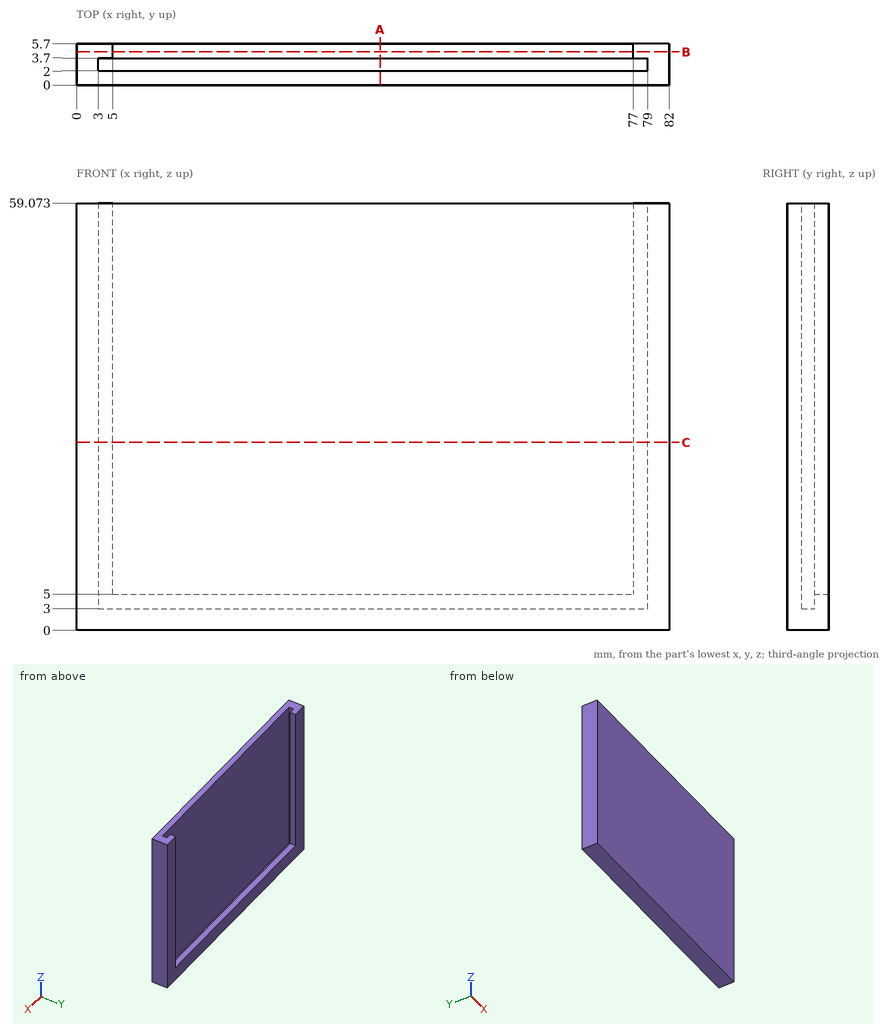
Input: dimensioned drawing with shaded views. Units: mm. Origin: part minimum x, y, z. Coordinates: 2 decimals unless noted, no trailing zeros. Order: outer loops, then holes, each group sorted by start corner. A loop starts at its lowest first (then second) coordinate and runs counter-clockwise, first axis right, second up. Notation, with made-up numbers: M -24,5.5 L -14,5.5 A25 cw -14,31.5 Z; hole C -22.75,57.25 d1. An arc over 180 degrees is marked long. Write each question's results on one line, items separated by ' | '. Start each with the question number.
Item 1: Cut plane A-A (x = 42). Return loops of the section in (y, z), and give its area (3 significant figures).
Item 2: Cut plane B-B (y = 4.6). Return loops of the section in (x, z).
Item 3: First-contact query: pin 1 Ø17 at (x, z) = (53.5, 26.5) entering from +Y; pin 2 Ø1.6 at (x, y) = (24, 5) entering from +Z. Flat tips, straight axial feed; report the tip coordinate or a pass-through.
Item 4: Cut plane C-C (z = 26). Return loops of the section in (x, y), and give its area (3 significant figures).
Item 5: Line query: probe 1 along X at (y, z) = (3.15, 51); probe 2 along X at (y, z) = (5, 30); probe 3 along Y at (x, z) = (5.5, 3.5). Output: solid intervals per line, ascending.
Checked values:
1) outline: M 0,0 L 5.7,0 L 5.7,5 L 3.7,5 L 3.7,3 L 2,3 L 2,59.07 L 0,59.07 Z | area: 133 mm2
2) outline: M 0,0 L 82,0 L 82,59.07 L 77,59.07 L 77,5 L 5,5 L 5,59.07 L 0,59.07 Z
3) pin 1: stops at y = 2 | pin 2: stops at z = 5
4) outline: M 0,0 L 82,0 L 82,5.7 L 77,5.7 L 77,3.7 L 79,3.7 L 79,2 L 3,2 L 3,3.7 L 5,3.7 L 5,5.7 L 0,5.7 Z | area: 194 mm2
5) probe 1: x = 0 to 3, 79 to 82 | probe 2: x = 0 to 5, 77 to 82 | probe 3: y = 0 to 2, 3.7 to 5.7
